Could you check a few things on this model? Use its own coordinates, in mm. Face numbers are marked on the shaded views. A direction names the side the tool comes from. Round coordinates to 2 decimals unless told otherwise and drop trailing zeros. Write each loop counter-clockwise with the first axis right and the second up, starting at its lowest first coordinate (ties: lowest second). Pieces come first, ordered by that corner, then holes. Notation, with made-up numbers: (61, 64.25) -> (109, 64.25) arc R26 ccw to (109, 89.25) -> close; hole circle Ø5 at (0.25, -12). An arc over 180 degrees is marked (long way). Answer in a Markdown table with one row per item. Add a question column.
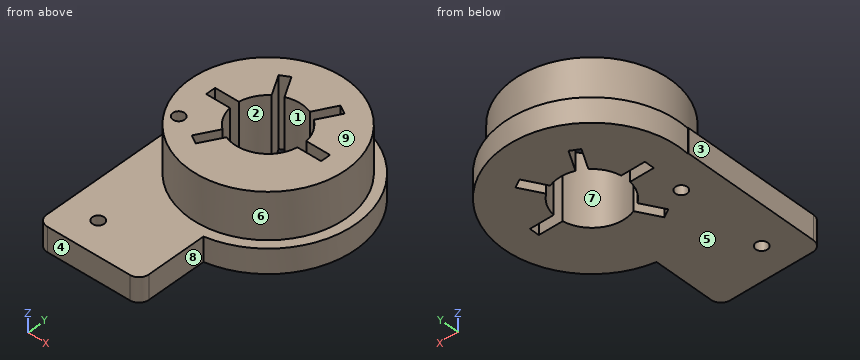
```python
from build123d import *

# Parameters (mm, degrees)
CYLINDER004_R     = 7
CYLINDER004_DEPTH = 20
BOX001_W          = 5
BOX001_H          = 2
BOX001_DEPTH      = 20
ARRAY006_COUNT    = 5
ARRAY006_ANGLE    = 240
CYLINDER014_R     = 1.2
CYLINDER014_DEPTH = 10
CYLINDER013_R     = 1.2
CYLINDER013_DEPTH = 20
CYLINDER006_R     = 16
CYLINDER006_DEPTH = 10
CYLINDER005_R     = 18
CYLINDER005_DEPTH = 5
BOX017_W          = 21
BOX017_H          = 30
BOX017_DEPTH      = 5
FILLET_R          = 2


with BuildPart() as cilindro004:
    # Cylinder004 → Cylinder004 (new body)
    with BuildSketch(Plane.XY):
        Circle(CYLINDER004_R)
    extrude(amount=CYLINDER004_DEPTH)


with BuildPart() as axle_model:
    # Box001 → Box001 (new body)
    with BuildSketch(Plane(origin=(6.8, -1, 0), x_dir=(1, 0, 0), z_dir=(0, 0, 1))):
        with Locations((2.5, 1)):
            Rectangle(BOX001_W, BOX001_H)
    extrude(amount=BOX001_DEPTH)

    # Array006: Axle_Model ×5 about axis
    array006_axis = Axis((0, 0, 0), (0, 0, 1))


with BuildPart() as axle_model_1:
    add(axle_model.part)
    for i in range(1, ARRAY006_COUNT):
        add(axle_model.part.rotate(array006_axis, i * ARRAY006_ANGLE / (ARRAY006_COUNT - 1)))

    # Fusion009: union Cilindro004
    add(cilindro004.part)


with BuildPart() as axle_model_2:
    # Fusion009 placement: moved
    add(axle_model_1.part.moved(Location((0, 0, 13))))


with BuildPart() as cilindro013:
    # Cylinder014 → Cylinder014 (new body)
    with BuildSketch(Plane(origin=(-11.3, -25.7, 14), x_dir=(1, 0, 0), z_dir=(0, 0, 1))):
        Circle(CYLINDER014_R)
    extrude(amount=CYLINDER014_DEPTH)


with BuildPart() as cilindro012:
    # Cylinder013 → Cylinder013 (new body)
    with BuildSketch(Plane(origin=(-11.3, -7.7, 14), x_dir=(1, 0, 0), z_dir=(0, 0, 1))):
        Circle(CYLINDER013_R)
    extrude(amount=CYLINDER013_DEPTH)


with BuildPart() as cilindro006:
    # Cylinder006 → Cylinder006 (new body)
    with BuildSketch(Plane.XY.offset(18)):
        Circle(CYLINDER006_R)
    extrude(amount=CYLINDER006_DEPTH)


with BuildPart() as fusion015:
    # Cylinder005 → Cylinder005 (new body)
    with BuildSketch(Plane.XY.offset(13.5)):
        Circle(CYLINDER005_R)
    extrude(amount=CYLINDER005_DEPTH)

    # Fusion015: union Cilindro006
    add(cilindro006.part)


with BuildPart() as sensorsupport:
    # Box017 → Box017 (new body)
    with BuildSketch(Plane(origin=(-18, -32, 13.5), x_dir=(1, 0, 0), z_dir=(0, 0, 1))):
        with Locations((10.5, 15)):
            Rectangle(BOX017_W, BOX017_H)
    extrude(amount=BOX017_DEPTH)

    # Fusion016: union Fusion015
    add(fusion015.part)


with BuildPart() as sensorsupport_1:
    # Fusion016 placement: moved
    add(sensorsupport.part.moved(Location((0, 0, 5))))

    # Cut015: cut Cilindro012
    add(cilindro012.part, mode=Mode.SUBTRACT)

    # Cut016: cut Cilindro013
    add(cilindro013.part, mode=Mode.SUBTRACT)

    # Cut: cut Axle_Model
    add(axle_model_2.part, mode=Mode.SUBTRACT)

    # Fillet
    fillet_edges = [sensorsupport_1.edges().sort_by_distance(p)[0] for p in [
        (-18, -32, 21),
        (3, -32, 21),
    ]]
    fillet(fillet_edges, radius=FILLET_R)


solid = sensorsupport_1.part
```
(1) If we mould it in two halves opening along Y, with no side actions, what happens to the marked faces 1, 2, 3 and 4? For each: pulls with the +Y half, pulls with the -Y half, needs draft (parallel to the pull), parting line crosses it, or undercut.
(2) For P1, Ø5.5, axis at y = -25.5, z = 20.5, coming from the +X side; P2, Ø4, axis at x = -9.5, z = 26.5, coming from the +Y side; P3, Ø1, axis at x = 11, z = 22, coming from the +Y side, each with a flat end and sliding along its axis, tell me the tip position at first contact or that it passes through.
(3) Suppose I cut it at A-A, the plane x = 0. Please give me the cut outline in (y, z).
(4) Suppose I cut it at D-D, the plane z = 22. State how many separate pieces and enclosed holes the cut face has, then the cut area to 3 significant figures.
(5) I need wall thicknesses on L1, parallel to X at y = -25.7, z = 19.8; L2, parallel to Y at x = -5.5, z = 19; L3, parallel to Y at x = -11.3, z = 22.75. Which ranges of each line are inside material? Lowest first, please.
(6) Suppose I cut it at B-B, the plane y = 0. Please give me the cut outline in (x, z).
(7) On a 3-axis mill with a long thin cutter (end or side, diameter ignored), from which of +Z, -Z, +X, -X, +Y, -Y can I reach the whole of each face in a straight line? I mean the marked faces 5, 6, 7, 8 and 9. Say none if no direction works.
(8) Suppose I cut it at C-C, the plane z = 30.25. Please give me the cut outline in (x, y), then the cut area to 3 significant figures.
Response:
| question | item | result |
|---|---|---|
| 1 | face 1 | undercut |
| 1 | face 2 | undercut |
| 1 | face 3 | needs draft |
| 1 | face 4 | pulls with the -Y half |
| 2 | P1 | x = 3 |
| 2 | P2 | y = 14.13 |
| 2 | P3 | y = 14.62 |
| 3 | outline | (-32, 18.5) -> (-7, 18.5) -> (-7, 33) -> (-16, 33) -> (-16, 23.5) -> (-32, 23.5) -> close; (7, 18.5) -> (18, 18.5) -> (18, 23.5) -> (16, 23.5) -> (16, 33) -> (7, 33) -> close |
| 4 | separate pieces | 1 |
| 4 | enclosed holes | 3 |
| 4 | area | 1,170 mm² |
| 5 | L1 | -18 to -12.5, -10.1 to 3 |
| 5 | L2 | -32 to -10.45, -7.53 to -4.33, 4.33 to 7.53, 10.45 to 17.14 |
| 5 | L3 | -32 to -26.9, -24.5 to -8.9, -6.5 to -1, 1 to 14.01 |
| 6 | outline | (-18, 18.5) -> (-11.8, 18.5) -> (-11.8, 33) -> (-16, 33) -> (-16, 23.5) -> (-18, 23.5) -> close; (11.8, 18.5) -> (18, 18.5) -> (18, 23.5) -> (16, 23.5) -> (16, 33) -> (11.8, 33) -> close |
| 7 | face 5 | -Z, +X, -X, +Y, -Y |
| 7 | face 6 | +Z |
| 7 | face 7 | +Z, -Z |
| 7 | face 8 | +Z, -Z, +X, -Y |
| 7 | face 9 | +Z, +X, -X, +Y, -Y |
| 8 | outline | circle Ø32 at (0, 0); hole circle Ø2.4 at (-11.3, -7.7); hole (-11.8, -1) -> (-6.93, -1) arc R7 ccw to (-4.33, -5.5) -> (-6.77, -9.72) -> (-5.03, -10.72) -> (-2.6, -6.5) arc R7 ccw to (6.93, -1) -> (11.8, -1) -> (11.8, 1) -> (6.93, 1) arc R7 ccw to (4.33, 5.5) -> (6.77, 9.72) -> (5.03, 10.72) -> (2.6, 6.5) arc R7 ccw to (-2.6, 6.5) -> (-5.03, 10.72) -> (-6.77, 9.72) -> (-4.33, 5.5) arc R7 ccw to (-6.93, 1) -> (-11.8, 1) -> close |
| 8 | area | 598 mm² |
